from build123d import *

# Parameters (mm, degrees)
SKETCH2_R          = 1
CUT_EXTRUDE1_DEPTH = 5
FILLET1_R          = 1.5
CHAMFER1_SIZE      = 0.25


with BuildPart() as part:
    # Sketch1 → Revolve1 (revolve)
    with BuildSketch(Plane.XY):
        Polygon((-49.42, 2.185), (-48.59, 2.185), (-48.5768767, 2.335), (-46.5768767, 2.335), (-46.563753401, 2.185), (47.4, 2.185), (47.4, 6.3), (50.8, 6.3), (50.8, 0), (-50.8, 0), (-50.8, 2.185), (-50.7868767, 2.335), (-49.7868767, 2.335), align=None)
    revolve(axis=Axis((-50.8, 0, 0), (1, 0, 0)))

    # Sketch2 → Cut-Extrude1 (cut)
    with BuildSketch(Plane(origin=(50.8, 0, 0), x_dir=(0, 0, -1), z_dir=(1, 0, 0))):
        Circle(SKETCH2_R)
    extrude(amount=-CUT_EXTRUDE1_DEPTH, mode=Mode.SUBTRACT)

    # Fillet1
    fillet1_edges = [part.edges().sort_by_distance(p)[0] for p in [
        (47.4, -6.3, 0),
        (50.8, -6.3, 0),
    ]]
    fillet(fillet1_edges, radius=FILLET1_R)

    # Chamfer1
    chamfer1_edges = [part.edges().sort_by_distance(p)[0] for p in [
        (50.8, 0, 1),
    ]]
    chamfer(chamfer1_edges, length=CHAMFER1_SIZE)


solid = part.part
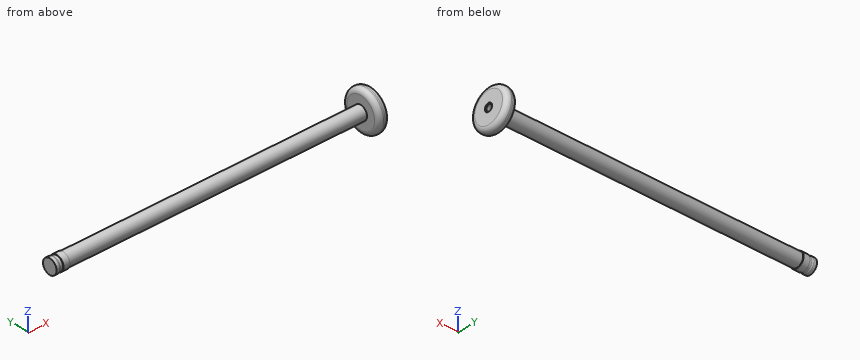
Input: part model. Units: mm. Frame: model coordinates. Give positions to 0.01 mm unless a question says otherwise; leave off trailing zeros. Order: outer loops, then holes, each group sorted by start corner. A loop starts at its lowest first (then second) coordinate and runs counter-clockwise, first axis right, second up. Notation, with made-up numbers: M 62.25,58 L 103.25,58 A33 ccw 103.25,93 Z; hole C 21,-5.5 d5. An arc over 180 degrees is marked long. Answer as a JSON object with one key per item and string values.
1. First-contact query: P1, Ø1.8, axis at y = 0, z = 0, coming from the +X side; P2, Ø5, axis at x = 22.5, y = -3.5, coming from the +Z side; P3, Ø4, axis at y = 4.5, z = -2.5, coming from the -X side; P4, Ø3, axis at y = -2, z = 1.5, coming from the -X side. Flat tips, straight axial feed; report the tip coordinate or a pass-through.
Result sheet:
{"P1": "x = 45.8", "P2": "z = 1.94", "P3": "x = 47.4", "P4": "x = -50.8"}
2. Cut plane C-C, the plane x = -27.5. Output: boundary loops of the cut face in (y, z) (3 decimals).
Result sheet:
{"outline": "C 0,0 d4.37"}
3. Ray query, line 1 (X direction, y = -2.5, z = -3.25); line 2 (Y direction, x = 3, z = 0.25); line 3 (Z direction, x = 34, y = 2). Return the intervals inside material, ascending. Write a range as [from, to].
Result sheet:
{"line 1": "[47.4, 50.8]", "line 2": "[-2.17, 2.17]", "line 3": "[-0.88, 0.88]"}
